Work out the finished part from the listing and answer in its coordinate system (mm). Coordinates: 2 decimals unless noted, no trailing zeros. Order: outer loops, then holes, each group sorted by start corner. A loop starts at its lowest first (then second) coordinate and runs counter-clockwise, first axis right, second up. Notation, with made-up numbers: (-29.75, -11) - (-13.75, -11) arc R15 ccw to (-13.75, 7) - close; hole circle Ø8 at (48, 39.5). An arc over 180 degrees is marked (long way). Answer as a JSON object with one key per item and string values. Group by question number.
1) Find the intervals of material crossed by line 1 along Y through (x, z) = (-12, -5); line 2 along Y through (x, z) = (-10.5, 3), in increasing order.
2) Section B-B (y = -19) is taken. Give the vertices of the cut face in (x, z).
3) Section A-A (x = -9.5) is taken. Give the vertices of the cut face in (y, z), plus the area to 3 significant figures.
4) Section C-C (z = 3.25) is taken. Give the vertices of the cut face in (x, y).
5) The mould has two halves that part along X. Classify faces 1 (the face through (-5.62, 20.79, -0.11)), 2 (the face through (-36.007, 0, 0)), 3 (the face through (-16, 1, 7.5)): released by +X, released by -X, zero draft, split by the parting line, or undercut.
from build123d import *

# Parameters (mm, degrees)
F0_W     = 40
F0_H     = 70
F0_R     = 3.5
F1_DEPTH = 7.5


with BuildPart() as f1:
    # F0 (on Top) → F1 (new body, symmetric)
    with BuildSketch(Plane.XY):
        with Locations((-16.007383, 0.540901)):
            Rectangle(F0_W, F0_H)
        with Locations((-8.853193, -17.868106)):
            Circle(F0_R, mode=Mode.SUBTRACT)
        with Locations((-8.853193, 22.131894)):
            Circle(F0_R, mode=Mode.SUBTRACT)
    extrude(amount=F1_DEPTH, both=True)


solid = f1.part
Report:
{
 "1": {"line 1": "y = -34.46 to -19.4, -16.34 to 20.6, 23.66 to 35.54", "line 2": "y = -34.46 to -20.96, -14.78 to 19.04, 25.22 to 35.54"},
 "2": {"outline": "(-36.01, -7.5) - (-12.17, -7.5) - (-12.17, 7.5) - (-36.01, 7.5) - close; (-5.54, -7.5) - (3.99, -7.5) - (3.99, 7.5) - (-5.54, 7.5) - close"},
 "3": {"outline": "(-34.46, -7.5) - (-21.31, -7.5) - (-21.31, 7.5) - (-34.46, 7.5) - close; (-14.43, -7.5) - (18.69, -7.5) - (18.69, 7.5) - (-14.43, 7.5) - close; (25.57, -7.5) - (35.54, -7.5) - (35.54, 7.5) - (25.57, 7.5) - close", "area": "844 mm²"},
 "4": {"outline": "(-36.01, -34.46) - (3.99, -34.46) - (3.99, 35.54) - (-36.01, 35.54) - close; hole circle Ø7 at (-8.85, -17.87); hole circle Ø7 at (-8.85, 22.13)"},
 "5": {"face 1": "undercut", "face 2": "released by -X", "face 3": "zero draft"}
}
